Read the model definition and answer for the solid it produces. Units are mm, in the model's axes. Face numbers are marked on the shaded views. Round coordinates to 2 decimals unless told otherwise and drop trailing zeros. Write each loop counter-clockwise with the first axis right and the second up, starting at its lowest first coordinate (ties: lowest second). Pieces come first, ordered by that corner, then holes.
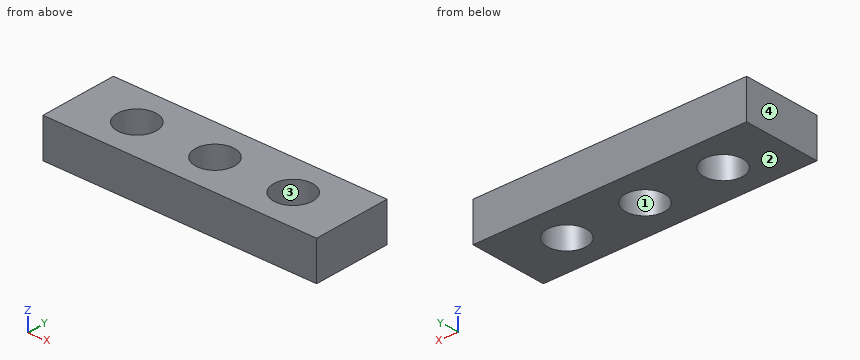
from build123d import *

# Parameters (mm, degrees)
SKETCH1_W           = 140
SKETCH1_H           = 40
SKETCH1_R           = 10
BOSS_EXTRUDE1_DEPTH = 20


with BuildPart() as part:
    # Sketch1 → Boss-Extrude1 (new body)
    with BuildSketch(Plane.XY):
        with Locations((70, 20)):
            Rectangle(SKETCH1_W, SKETCH1_H)
        with Locations((30, 20)):
            Circle(SKETCH1_R, mode=Mode.SUBTRACT)
        with Locations((70, 20)):
            Circle(SKETCH1_R, mode=Mode.SUBTRACT)
        with Locations((110, 20)):
            Circle(SKETCH1_R, mode=Mode.SUBTRACT)
    extrude(amount=-BOSS_EXTRUDE1_DEPTH)


solid = part.part
Q1. Determine the mould class of the marked faces 1, 2, 3 and 4 for opening direction X: pulls with the +X half, pulls with the -X half, needs draft (parallel to the pull), parting line crosses it, or undercut.
Verdict:
face 1: undercut
face 2: needs draft
face 3: undercut
face 4: pulls with the -X half
Q2. Straight lines are drawn through the part: probe 1 along Y at (x, z) = (70, -14.25); probe 2 along X at (y, z) = (18, -9.75); probe 3 along Y at (x, z) = (69, -16.5). For each, find the intervals that lie inside material, in ascending order.
Verdict:
probe 1: y = 0 to 10, 30 to 40
probe 2: x = 0 to 20.2, 39.8 to 60.2, 79.8 to 100.2, 119.8 to 140
probe 3: y = 0 to 10.05, 29.95 to 40
Q3. Section C-C (y = 26) is taken. Determine the outline of the cut face in (x, z).
Verdict:
outline: (0, -20) - (22, -20) - (22, 0) - (0, 0) - close; (38, -20) - (62, -20) - (62, 0) - (38, 0) - close; (78, -20) - (102, -20) - (102, 0) - (78, 0) - close; (118, -20) - (140, -20) - (140, 0) - (118, 0) - close
Q4. Section B-B (z = -3.5) is taken. Determine the outline of the cut face in (x, y), then the cut area to 3 significant figures.
Verdict:
outline: (0, 0) - (140, 0) - (140, 40) - (0, 40) - close; hole circle Ø20 at (30, 20); hole circle Ø20 at (70, 20); hole circle Ø20 at (110, 20)
area: 4,660 mm2
Q5. Section D-D (x = 29) is taken. Determine the outline of the cut face in (y, z).
Verdict:
outline: (0, -20) - (10.05, -20) - (10.05, 0) - (0, 0) - close; (29.95, -20) - (40, -20) - (40, 0) - (29.95, 0) - close
Q6. A flat-ended cylindrical pin translates along its axis: pin 1 Ø10 at (x, y) = (14, 15) entering from +Z. Find the tip coordinate at first contact, or state that the pin passes through.
Verdict:
pin 1: stops at z = 0
Q7. Section A-A (x = 70) is taken. Determine the outline of the cut face in (y, z).
Verdict:
outline: (0, -20) - (10, -20) - (10, 0) - (0, 0) - close; (30, -20) - (40, -20) - (40, 0) - (30, 0) - close
